from build123d import *

# Parameters (mm, degrees)
SKETCH1_W           = 79.756
SKETCH1_H           = 7.62
BOSS_EXTRUDE1_DEPTH = 8.89
SKETCH2_W           = 8.89
SKETCH2_H           = 7.62
CUT_EXTRUDE1_DEPTH  = 6.35
SKETCH3_W           = 8.89
SKETCH3_H           = 7.62
CUT_EXTRUDE2_DEPTH  = 6.35
SKETCH4_W           = 54.9148
SKETCH4_H           = 7.62
CUT_EXTRUDE3_DEPTH  = 7.366
SKETCH5_W           = 4.064
SKETCH5_H           = 5.461
CUT_EXTRUDE4_DEPTH  = 1.524
SKETCH7_W           = 3.683
SKETCH7_H           = 4.445
BOSS_EXTRUDE2_DEPTH = 1.524
SKETCH8_R           = 2.1717
CUT_EXTRUDE5_DEPTH  = 2.54
SKETCH9_R           = 2.1717
CUT_EXTRUDE6_DEPTH  = 2.54


with BuildPart() as part:
    # Sketch1 → Boss-Extrude1 (new body)
    with BuildSketch(Plane(origin=(0, 0, 0), x_dir=(1, 0, 0), z_dir=(0, 1, 0))):
        with Locations((25.937163647, -9.682646588)):
            Rectangle(SKETCH1_W, SKETCH1_H)
    extrude(amount=BOSS_EXTRUDE1_DEPTH)

    # Sketch2 → Cut-Extrude1 (cut)
    with BuildSketch(Plane(origin=(0, 8.89, 0), x_dir=(1, 0, 0), z_dir=(0, 1, 0))):
        with Locations((-9.495836353, -9.682646588)):
            Rectangle(SKETCH2_W, SKETCH2_H)
    extrude(amount=-CUT_EXTRUDE1_DEPTH, mode=Mode.SUBTRACT)

    # Sketch3 → Cut-Extrude2 (cut)
    with BuildSketch(Plane(origin=(0, 8.89, 0), x_dir=(1, 0, 0), z_dir=(0, 1, 0))):
        with Locations((61.370163647, -9.682646588)):
            Rectangle(SKETCH3_W, SKETCH3_H)
    extrude(amount=-CUT_EXTRUDE2_DEPTH, mode=Mode.SUBTRACT)

    # Sketch4 → Cut-Extrude3 (cut)
    with BuildSketch(Plane(origin=(0, 8.89, 0), x_dir=(1, 0, 0), z_dir=(0, 1, 0))):
        with Locations((26.216563647, -9.682646588)):
            Rectangle(SKETCH4_W, SKETCH4_H)
    extrude(amount=-CUT_EXTRUDE3_DEPTH, mode=Mode.SUBTRACT)

    # Sketch5 → Cut-Extrude4 (cut)
    with BuildSketch(Plane(origin=(-1.240836353, 0, 0), x_dir=(0, 0, -1), z_dir=(1, 0, 0))):
        with Locations((-9.682646588, 4.2545)):
            Rectangle(SKETCH5_W, SKETCH5_H)
    extrude(amount=-CUT_EXTRUDE4_DEPTH, mode=Mode.SUBTRACT)

    # Sketch7 → Boss-Extrude2 (add)
    with BuildSketch(Plane.ZY.offset(-53.673963647)):
        with Locations((9.682646588, 4.7625)):
            Rectangle(SKETCH7_W, SKETCH7_H)
    extrude(amount=BOSS_EXTRUDE2_DEPTH)

    # Sketch8 → Cut-Extrude5 (cut)
    with BuildSketch(Plane(origin=(0, 2.54, 0), x_dir=(1, 0, 0), z_dir=(0, 1, 0))):
        with Locations(Location((-9.495836353, -9.682646588, 0), (0, 0, 270))):
            Circle(SKETCH8_R)
    extrude(amount=-CUT_EXTRUDE5_DEPTH, mode=Mode.SUBTRACT)

    # Sketch9 → Cut-Extrude6 (cut)
    with BuildSketch(Plane(origin=(0, 2.54, 0), x_dir=(1, 0, 0), z_dir=(0, 1, 0))):
        with Locations(Location((61.370163647, -9.682646588, 0), (0, 0, 270))):
            Circle(SKETCH9_R)
    extrude(amount=-CUT_EXTRUDE6_DEPTH, mode=Mode.SUBTRACT)


solid = part.part
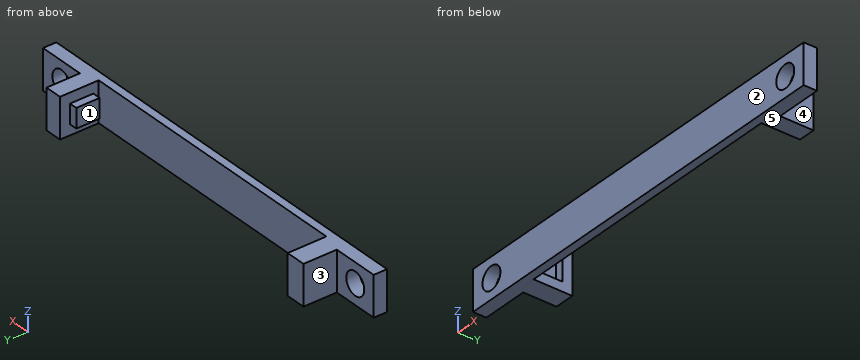
Work out the finished part from the listing and answer in its coordinate system (mm). Face numbers are marked on the shaded views. A direction names the side the tool comes from. Give positions to 0.01 mm unless a question says otherwise; leave off trailing zeros. Loops run counter-clockwise (first coordinate to the right, second up) from the corner with the lowest first, then second, coordinate; pieces in that order, holes last. Notation, with made-up numbers: (61.5, -14.75) - (79.5, -14.75) arc R30 cw to (79.5, 7.25) - close; hole circle Ø9 at (-5.5, 32). An arc over 180 degrees is marked (long way). Answer in a Markdown table with one row per item.
(1) A tool of negligible diameter and unlimited length cuts with its end or side. For the marked faces 4 and 5, from which of +Z, -Z, +X, -X, +Y, -Y can it reach the whole face along a straight path? Write none if from no direction.
Results list:
| item | result |
|---|---|
| face 4 | +Z, -Z, +X, +Y |
| face 5 | -Z, +X, -X, +Y, -Y |
(2) Section A-A (y = 6.25) is taken. Give the vertices of the cut face in (x, z), and give its area (3 significant figures).
Results list:
| item | result |
|---|---|
| outline | (-5.05, 5.87) - (-1.24, 5.87) - (-1.24, 7.65) - (-2.76, 7.65) - (-2.76, 11.71) - (-1.24, 11.71) - (-1.24, 13.49) - (-5.05, 13.49) - close; (52.15, 7.84) - (53.67, 7.84) - (53.67, 5.87) - (56.93, 5.87) - (56.93, 13.49) - (53.67, 13.49) - (53.67, 11.52) - (52.15, 11.52) - close |
| area | 53.2 mm² |
(3) For a pull along X with two mould halves and no side action, classify the marked faces 1, 2 and 3 as pulls with the +X half, pulls with the -X half, needs draft (parallel to the pull), parting line crosses it, or undercut.
Results list:
| item | result |
|---|---|
| face 1 | undercut |
| face 2 | needs draft |
| face 3 | pulls with the -X half |
(4) Consider L1, parallel to X at y = 4.75, z = 12.5; L2, parallel to X at y = 6.75, z = 10.5; L3, parallel to X at y = 1, z = 7.75. Determine where each line is inside the solid, lowest interval first. Write a range as [from, to].
Results list:
| item | result |
|---|---|
| L1 | x = [-5.05, -1.24], [53.67, 56.93] |
| L2 | x = [-5.05, -2.76], [52.15, 56.93] |
| L3 | x = [-13.94, -10.49], [-8.51, 60.38], [62.36, 65.82] |
(5) Section C-C (x = -8) is taken. Give the vertices of the cut face in (y, z).
Results list:
| item | result |
|---|---|
| outline | (0, 5.87) - (2.54, 5.87) - (2.54, 8.11) - (0, 8.11) - close; (0, 11.26) - (2.54, 11.26) - (2.54, 13.49) - (0, 13.49) - close |
(6) Section D-D (z = 6.75) is taken. Give the vertices of the cut face in (x, y).
Results list:
| item | result |
|---|---|
| outline | (-13.94, 0) - (65.82, 0) - (65.82, 2.54) - (56.93, 2.54) - (56.93, 8.89) - (53.67, 8.89) - (53.67, 1.52) - (-1.24, 1.52) - (-1.24, 8.89) - (-5.05, 8.89) - (-5.05, 2.54) - (-13.94, 2.54) - close |
(7) Section B-B (z = 10) is taken. Give the vertices of the cut face in (x, y) (3 decimals), and give its area (3 significant figures).
Results list:
| item | result |
|---|---|
| outline | (-13.941, 0) - (-11.644, 0) - (-11.644, 2.54) - (-13.941, 2.54) - close; (-7.347, 0) - (59.222, 0) - (59.222, 2.54) - (56.925, 2.54) - (56.925, 8.89) - (53.674, 8.89) - (53.674, 6.985) - (52.15, 6.985) - (52.15, 2.54) - (53.674, 2.54) - (53.674, 1.524) - (-2.765, 1.524) - (-2.765, 6.985) - (-1.241, 6.985) - (-1.241, 8.89) - (-5.051, 8.89) - (-5.051, 2.54) - (-7.347, 2.54) - close; (63.519, 0) - (65.815, 0) - (65.815, 2.54) - (63.519, 2.54) - close |
| area | 168 mm² |
(8) Flat-ended cylindrical pins translate along their axes: pin 1 Ø1.5 at (y, z) = (7, 10.5) entering from -X; pin 2 Ø3 at (y, z) = (4.5, 9) entering from +X; pin 3 Ø2.5 at (x, z) = (62.5, 9.5) entering from +Y. Find the tip coordinate at first contact, or state that the pin passes through.
Results list:
| item | result |
|---|---|
| pin 1 | stops at x = -5.05 |
| pin 2 | stops at x = 56.93 |
| pin 3 | stops at y = 2.54 |
